Part print with two shaded views. Sizes in mm from the minimum x, y, z corner. Give positions to 0.01 mm unless a question says otherwise; leave off trailing zeros. Write each loop counter-clockwise with the first axis right and the second up, starting at its lowest first coordinate (ties: lowest second). Pieces come first, ordered by that corner, then holes.
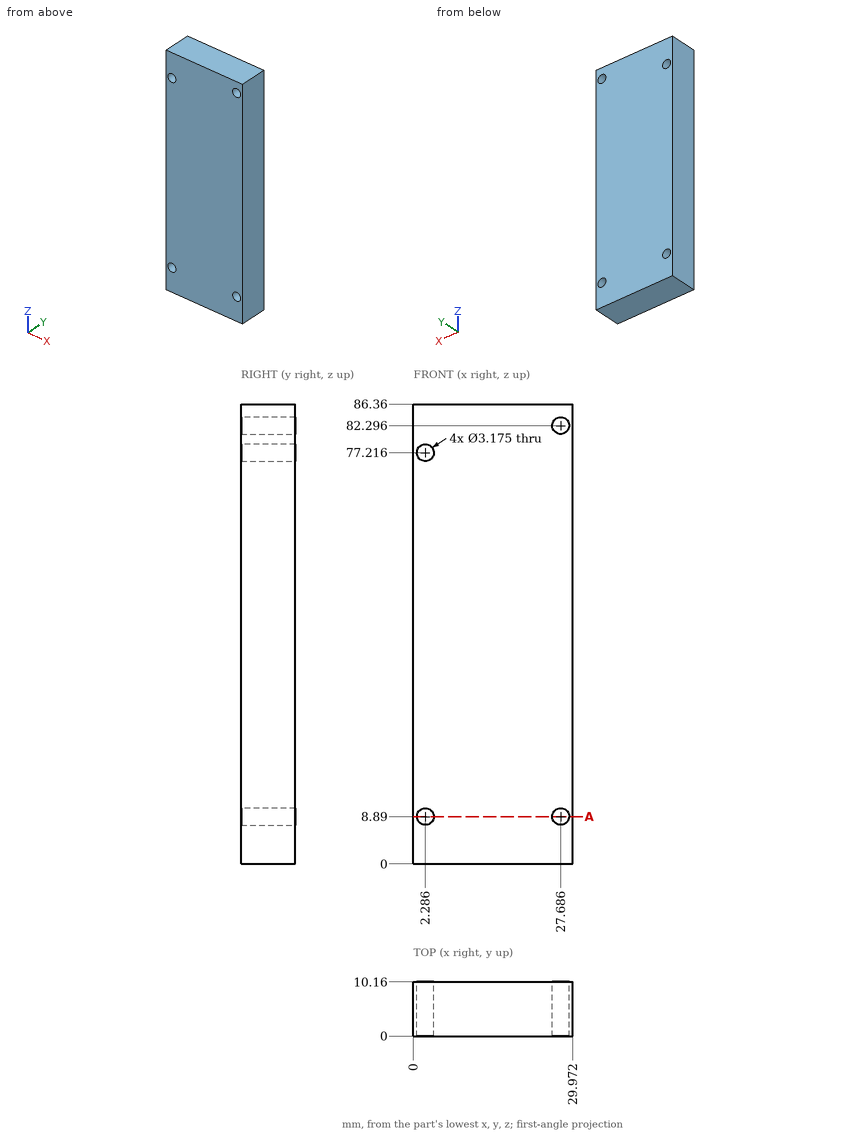
1) Saw through at A-A, the plane z = 8.89. Write the cut outline in (x, y).
Answers follow:
outline: (0, 0) - (0.7, 0) - (0.7, 10.16) - (0, 10.16) - close; (3.87, 0) - (26.1, 0) - (26.1, 10.16) - (3.87, 10.16) - close; (29.27, 0) - (29.97, 0) - (29.97, 10.16) - (29.27, 10.16) - close
2) Wall check: L1, parallel to X at y = 2.5, z = 8.89; L2, parallel to Z at x = 2.75, y = 9.5; L3, parallel to Z at x = 2, y = 8.5. Give the ranges that are in metal, low to high.
Answers follow:
L1: x = 0 to 0.7, 3.87 to 26.1, 29.27 to 29.97
L2: z = 0 to 7.37, 10.41 to 75.7, 78.73 to 86.36
L3: z = 0 to 7.33, 10.45 to 75.65, 78.78 to 86.36
3) Pin check, flat tip, straight feed: pin 1 Ø1.9 at (x, z) = (2.286, 77.216) entering from +Y. Stop position of the tip, or through.
Answers follow:
pin 1: passes through
